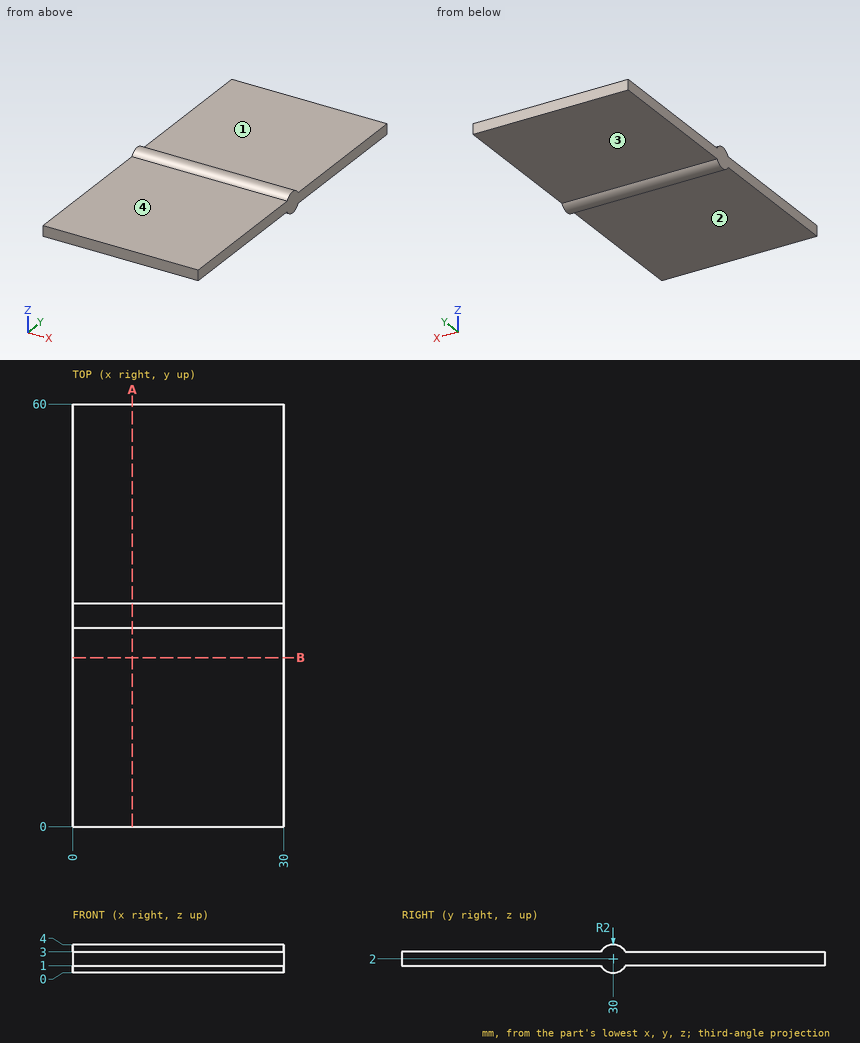
The drawing under review shows one solid part. Ordinate dimensions are in mm from its lowest x, y, z. A direction names the side the tool comes from. Give positions to 0.01 mm unless a question says otherwise; leave off trailing zeros. Order: outer loops, then holes, each group sorted by start corner. A loop starts at its lowest first (then second) coordinate and runs counter-clockwise, first axis right, second up. Notation, with made-up numbers: (4.25, -31) -> (19.25, -31) arc R38 cw to (19.25, 7) -> close; hole circle Ø9 at (37, 19.5). An arc over 180 degrees is marked (long way). Write item = value, one per line.
1) To check wall thickness, follow L1, parallel to Z at x = 13, y = 4; L2, parallel to Z at x = 27, y = 29.5; L3, parallel to Y at x = 25.25, z = 0.4. State the ranges of each line that lie inside material, in increasing order. Write a range as from..to.
Findings:
L1 = 1..3
L2 = 0.06..3.94
L3 = 28.8..31.2
2) We need section B-B, the plane y = 24. Give the boundary of the cut face in (x, z), and give its area (3 significant figures).
Findings:
outline = (0, 1) -> (30, 1) -> (30, 3) -> (0, 3) -> close
area = 60.0 mm^2
3) For the marked faces 1, 2, 3 and 4, list the 3-axis set-ups (+Z, -Z, +X, -X, +Y, -Y) from which the entire face can be reached by the end or side of a thin tool; tool diameter is ignored.
Findings:
face_1 = +Z, +X, -X, +Y
face_2 = -Z, +X, -X, -Y
face_3 = -Z, +X, -X, +Y
face_4 = +Z, +X, -X, -Y
4) Insertion check: pin 1 (12 mm diameter, centred on x = 5.5, y = 20, fed in from -Z); pin 2 (3 mm diameter, centred on x = 4.5, y = 35.5, fed in from +Z). Each pin has a flat end and moves straight along its axis. Give the tip position at first contact, or say it passes through.
Findings:
pin_1 = 1
pin_2 = 3
5) We need section A-A, the plane x = 8.5. Give the boundary of the cut face in (y, z).
Findings:
outline = (0, 1) -> (28.27, 1) arc R2 ccw to (31.73, 1) -> (60, 1) -> (60, 3) -> (31.73, 3) arc R2 ccw to (28.27, 3) -> (0, 3) -> close
